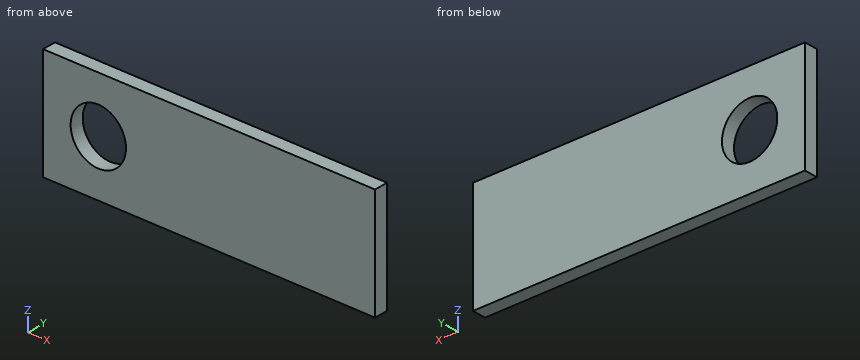
Autodesk Inventor part; units mm, degrees
ref_plane "YZ Plane" through (0, 0, 0) normal (1, 0, 0) x (0, 1, 0)
ref_plane "XZ Plane" through (0, 0, 0) normal (0, 1, 0) x (-1, 0, 0)
ref_plane "XY Plane" through (0, 0, 0) normal (0, 0, 1) x (1, 0, 0)
sketch "Sketch1" plane through (0, 0, 0) normal (0, 1, 0) x (-1, 0, 0)
  line L0 (-76.2, -12.7) -> (76.2, -12.7)
  line L1 (76.2, -12.7) -> (76.2, 12.7)
  line L2 (76.2, 12.7) -> (-76.2, 12.7)
  line L3 (-76.2, 12.7) -> (-76.2, -12.7)
  line L4 (-76.2, -12.7) -> (76.2, 12.7) construction
  line L5 (76.2, -12.7) -> (-76.2, 12.7) construction
  line L6 (-76.2, 0) -> (-63.5, 0)
  line L7 (-76.2, 0) -> (-63.5, 0) construction
  line L8 (76.2, 0) -> (50.8, 0)
  line L9 (76.2, 0) -> (101.6, 0) construction
  line L10 (50.8, 0) -> (25.4, 0)
  circle A0 centre (-63.5, 0) radius 3.175
  circle A1 centre (25.4, 0) radius 3.175
  point P0 (0, 0)
  dimension "d0" = 152.4
  dimension "d1" = 25.4
  dimension "d2" = 12.7
  dimension "d3" = 0
  dimension "d4" = 25.4
  dimension "d5" = 180
  dimension "d6" = 25.4
  dimension "d7" = 6.35
  dimension "d8" = 6.35
extrude "Extrusion1" add sketch "Sketch1" along normal blind 3.175
sketch "Sketch2" plane through (0, 3.175, 0) normal (0, 1, 0) x (1, 0, 0)
  circle A0 centre (-63.5, 0) radius 3.175
  point P0 (0, 0)
  dimension "d11" = 6.35
extrude "Extrusion2" cut sketch "Sketch2" against normal blind 25.4
sketch "Sketch3" plane through (0, 3.175, 0) normal (0, 1, 0) x (1, 0, 0)
  circle A0 centre (-63.5, 0) radius 3.175
  circle A1 centre (-63.5, 0) radius 6.35
  point P0 (0, 0)
  dimension "d14" = 12.7
extrude "Extrusion3" cut sketch "Sketch3" against normal blind 25.4
sketch "Sketch4" plane through (0, 3.175, 0) normal (0, 1, 0) x (1, 0, 0)
  circle A0 centre (63.5, 0) radius 3.175
  line L0 (76.2, 12.7) -> (-76.2, 12.7)
  line L1 (-76.2, -12.7) -> (76.2, -12.7)
  line L2 (76.2, -12.7) -> (76.2, 12.7)
  line L3 (0, 12.7) -> (0, -12.7)
  point P0 (0, 0)
extrude "Extrusion4" cut sketch "Sketch4" against normal blind 25.4
sketch "Sketch5" plane through (0, 3.175, 0) normal (0, 1, 0) x (1, 0, 0)
  circle A0 centre (-25.4, 0) radius 3.175
  circle A1 centre (-25.4, 0) radius 3.175
  point P0 (0, 0)
extrude "Extrusion5" add sketch "Sketch5" against normal blind 3.175
properties part number "BarHolder"
Build history of the part. All positions in model axes, mm. Coordinates: 2 decimals unless noted, no trailing zeros. Order: outer loops, then holes, each group sorted by start corner. A loop starts at its lowest first (then second) coordinate and runs counter-clockwise, first axis right, second up.
Item 1: Saw through at C-C on y = 2.6. List the corners of the cut face in (x, z), then the cut area to 3 significant figures.
Filled in:
outline: (-76.2, -12.7) - (0, -12.7) - (0, 12.7) - (-76.2, 12.7) - close; hole circle Ø12.7 at (-63.5, 0)
area: 1,810 mm2
Item 2: Drop flat-ended pins along their axis: pin 1 Ø1 at (y, z) = (2, -7) entering from +X; pin 2 Ø10 at (x, z) = (-63.5, 0) entering from -Y. Give the stop position or say it passes through.
Filled in:
pin 1: stops at x = 0
pin 2: passes through
Item 3: Saw through at A-A on z = 0. List the corners of the cut face in (x, y) (3 decimals), then the cut area to 3 significant figures.
Filled in:
outline: (-76.2, 0) - (-69.85, 0) - (-69.85, 3.175) - (-76.2, 3.175) - close; (-57.15, 0) - (0, 0) - (0, 3.175) - (-57.15, 3.175) - close
area: 202 mm2
Item 4: Drill centre lines: L1, parallel to X at y = 1.65, z = 0; L2, parallel to Z at x = -63.5, y = 2.3; L3, parallel to X at y = 1.9, z = 2.5. Where is each one in solid material? Low to high.
Filled in:
L1: x = -76.2 to -69.85, -57.15 to 0
L2: z = -12.7 to -6.35, 6.35 to 12.7
L3: x = -76.2 to -69.34, -57.66 to 0
Item 5: Saw through at B-B on x = -63.5. List the corners of the cut face in (y, z) (3 decimals), then the cut area to 3 significant figures.
Filled in:
outline: (0, -12.7) - (3.175, -12.7) - (3.175, -6.35) - (0, -6.35) - close; (0, 6.35) - (3.175, 6.35) - (3.175, 12.7) - (0, 12.7) - close
area: 40.3 mm2
